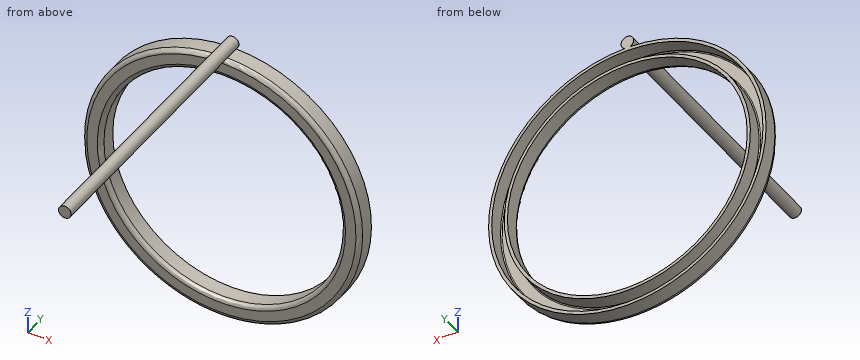
from build123d import *

# Parameters (mm, degrees)
EXTRUDE1_DEPTH      = 0.9
EXTRUDE1_DEPTH_BACK = 12.5
SKETCH3_R           = 0.3


with BuildPart() as part:
    # Sketch1 → Revolve-Thin1 (revolve)
    with BuildSketch(Plane.XY, mode=Mode.PRIVATE) as revolve_thin1_sk:
        with BuildLine():
            Line((-6.625, 0.9), (-6.625, 0.2))
            ThreePointArc((-6.625, 0.2), (-6.566421356, 0.058578644), (-6.425, 0))
            Line((-6.425, 0), (-5.925, 0))
            ThreePointArc((-5.925, 0), (-5.783578644, 0.058578644), (-5.725, 0.2))
            Line((-5.725, 0.2), (-5.725, 0.9))
            Line((-5.725, 0.9), (-5.875, 0.9))
            Line((-5.875, 0.9), (-5.875, 0.2))
            ThreePointArc((-5.875, 0.2), (-5.889644661, 0.164644661), (-5.925, 0.15))
            Line((-5.925, 0.15), (-6.425, 0.15))
            ThreePointArc((-6.425, 0.15), (-6.460355339, 0.164644661), (-6.475, 0.2))
            Line((-6.475, 0.2), (-6.475, 0.9))
            Line((-6.475, 0.9), (-6.625, 0.9))
        make_face()
    revolve(revolve_thin1_sk.sketch.rotate(Axis((0, 22.559206249, 0), (0, -1, 0)), 270), axis=Axis((0, 22.559206249, 0), (0, -1, 0)))

    # Sketch3 → Extrude1 (add, two sides: drawn at the far end of the back side and taken through both)
    with BuildSketch(Plane(origin=(0, 0, 0), x_dir=(1, 0, 0), z_dir=(0, 1, 0)).offset(-EXTRUDE1_DEPTH_BACK)):
        with Locations(Location((0, -6.9, 0), (0, 0, 270))):
            Circle(SKETCH3_R)
    extrude(amount=EXTRUDE1_DEPTH + EXTRUDE1_DEPTH_BACK)


solid = part.part
Can you work these out from the model? Positions are in its coordinate system, mm. Coordinates: 2 decimals unless noted, no trailing zeros. Write each loop counter-clockwise with the first axis right and the second up, starting at its lowest first coordinate (ties: lowest second). Pieces come first, ordered by that corner, then holes. Notation, with made-up numbers: (38.25, 33.25) -> (82.25, 33.25) arc R27 cw to (82.25, 60.25) -> close; hole circle Ø2 at (-29.5, 83). An arc over 180 degrees is marked (long way). Write each question's results on one line, items separated by ' | '. Start each with the question number.
Item 1: If we section it at C-C, the plane z = 6.9: Write out the boundary of the cut face in (x, y).
Item 2: Please list where these lines run through material, in increasing order: probe 1 along X at (y, z) = (-2.75, 6.75); probe 2 along Y at (x, z) = (4.5, 4.75).
Item 3: If we section it at B-B, the plane y = -4: Write out the boundary of the cut face in (x, z), and give its area (3 significant figures).
Item 4: I'm going to push flat-ended pins straight in: P1, Ø8, axis at y = -7.5, z = 3, coming from the -X side; P2, Ø6, axis at x = -2, z = -4, coming from the +Y side. Where does each tip first touch, or does it pass through?
Item 5: If we section it at A-A, the plane z = 0: Write out the boundary of the cut face in (x, y) (3 decimals).
Answer block:
1) outline: (-0.3, -12.5) -> (0.3, -12.5) -> (0.3, 0.9) -> (-0.3, 0.9) -> close
2) probe 1: -0.26 to 0.26 | probe 2: 0.04 to 0.9
3) outline: circle Ø0.6 at (0, 6.9) | area: 0.283 mm²
4) P1: x = -0.3 | P2: y = 0.9
5) outline: (-6.625, 0.2) arc R0.2 ccw to (-6.425, 0) -> (-5.925, 0) arc R0.2 ccw to (-5.725, 0.2) -> (-5.725, 0.9) -> (-5.875, 0.9) -> (-5.875, 0.2) arc R0.05 cw to (-5.925, 0.15) -> (-6.425, 0.15) arc R0.05 cw to (-6.475, 0.2) -> (-6.475, 0.9) -> (-6.625, 0.9) -> close; (5.725, 0.2) arc R0.2 ccw to (5.925, 0) -> (6.425, 0) arc R0.2 ccw to (6.625, 0.2) -> (6.625, 0.9) -> (6.475, 0.9) -> (6.475, 0.2) arc R0.05 cw to (6.425, 0.15) -> (5.925, 0.15) arc R0.05 cw to (5.875, 0.2) -> (5.875, 0.9) -> (5.725, 0.9) -> close
